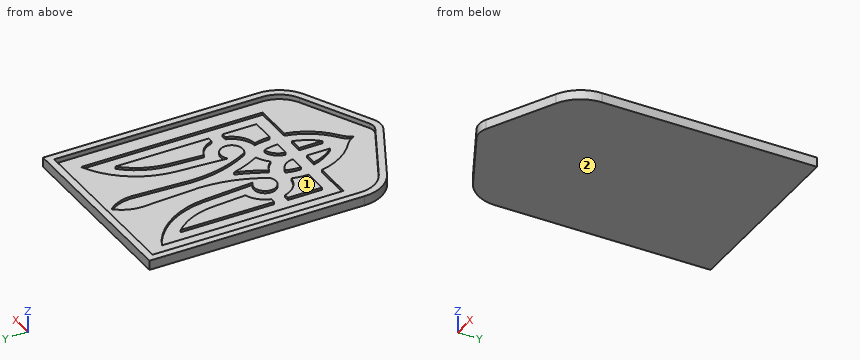
from build123d import *

# Parameters (mm, degrees)
EXTRUDE_1_DEPTH     = 2
EXTRUDE_2_DEPTH     = 2
OTHER_START         = 1
OTHER_1_DEPTH       = 1
CUT_EXTRUDE_1_DEPTH = 10


# Read off the part's stored shape, not the designer's step: Полость1
with BuildPart() as part:
    # Эскиз1 → Бобышка-Вытянуть1 (new body)
    with BuildSketch(Plane.XY):
        with BuildLine():
            Line((-3.59812982, 1.811928513), (-31.19625964, 15.709658955))
            ThreePointArc((-31.19625964, 15.709658955), (-37.622410841, 21.607746257), (-40, 30))
            Line((-40, 30), (-40, 120))
            Line((-40, 120), (40, 120))
            Line((40, 120), (40, 30))
            ThreePointArc((40, 30), (37.622410841, 21.607746257), (31.19625964, 15.709658955))
            Line((31.19625964, 15.709658955), (3.59812982, 1.811928513))
            ThreePointArc((3.59812982, 1.811928513), (0, 0.957099036), (-3.59812982, 1.811928513))
        make_face()
    extrude(amount=EXTRUDE_1_DEPTH)

    # Эскиз2 → Бобышка-Вытянуть2 (add)
    with BuildSketch(Plane.XY.offset(2)):
        with BuildLine():
            Line((40, 120), (-40, 120))
            Line((-40, 120), (-40, 30))
            ThreePointArc((-40, 30), (-37.622410841, 21.607746257), (-31.19625964, 15.709658955))
            Line((-31.19625964, 15.709658955), (-3.59812982, 1.811928513))
            ThreePointArc((-3.59812982, 1.811928513), (0, 0.957099036), (3.59812982, 1.811928513))
            Line((3.59812982, 1.811928513), (31.19625964, 15.709658955))
            ThreePointArc((31.19625964, 15.709658955), (37.622410841, 21.607746257), (40, 30))
            Line((40, 30), (40, 120))
        make_face()
        with BuildLine():
            Line((37, 117), (-37, 117))
            Line((-37, 117), (-37, 30))
            ThreePointArc((-37, 30), (-35.068208808, 23.181293834), (-29.846960958, 18.389097901))
            Line((-29.846960958, 18.389097901), (-2.248831138, 4.491367459))
            ThreePointArc((-2.248831138, 4.491367459), (0, 3.957099036), (2.248831138, 4.491367459))
            Line((2.248831138, 4.491367459), (29.846960958, 18.389097901))
            ThreePointArc((29.846960958, 18.389097901), (35.068208808, 23.181293834), (37, 30))
            Line((37, 30), (37, 117))
        make_face(mode=Mode.SUBTRACT)
    extrude(amount=EXTRUDE_2_DEPTH)

    # Полость1 outline → Полость1 (cut)
    with BuildSketch(Plane.XY.offset(OTHER_START)):
        with BuildLine():
            ThreePointArc((9.788029472, 60.549586915), (17.495233568, 56.130696454), (9.431968209, 52.400905625))
            ThreePointArc((9.431968209, 52.400905625), (4.262579544, 64.984556644), (2.5, 78.473966026))
            Line((2.5, 78.473966026), (3.75, 103.098966026))
            ThreePointArc((3.75, 103.098966026), (2.7812152, 108.402266884), (0, 113.020533442))
            ThreePointArc((0, 113.020533442), (-2.7812152, 108.402266884), (-3.75, 103.098966026))
            Line((-3.75, 103.098966026), (-2.5, 78.473966026))
            ThreePointArc((-2.5, 78.473966026), (-4.262579544, 64.984556644), (-9.431968209, 52.400905625))
            ThreePointArc((-9.431968209, 52.400905625), (-17.495233567, 56.130696454), (-9.788029472, 60.549586915))
            Line((-9.788029472, 60.549586915), (-11.224736233, 81.095450805))
            ThreePointArc((-11.224736233, 81.095450805), (-16.940759264, 97.456053222), (-30, 108.848966026))
            Line((-30, 108.848966026), (-30, 33.848966026))
            Line((-30, 33.848966026), (-13.791634566, 33.848966026))
            ThreePointArc((-13.791634566, 33.848966026), (-10.030008845, 24.210277963), (-2.972883984, 16.643830691))
            ThreePointArc((-2.972883984, 16.643830691), (-1.271172874, 15.008808512), (0, 13.020533442))
            ThreePointArc((0, 13.020533442), (1.271172874, 15.008808512), (2.972883984, 16.643830691))
            ThreePointArc((2.972883984, 16.643830691), (10.030008845, 24.210277963), (13.791634566, 33.848966026))
            Line((13.791634566, 33.848966026), (30, 33.848966026))
            Line((30, 33.848966026), (30, 108.848966026))
            ThreePointArc((30, 108.848966026), (16.940759264, 97.456053222), (11.224736233, 81.095450805))
            Line((11.224736233, 81.095450805), (9.788029472, 60.549586915))
        make_face()
        with BuildLine():
            ThreePointArc((-2.5, 22.780752061), (-6.389541147, 27.869966821), (-8.687410968, 33.848966026))
            Line((-8.687410968, 33.848966026), (-2.5, 33.848966026))
            Line((-2.5, 33.848966026), (-2.5, 22.780752061))
        make_face(mode=Mode.SUBTRACT)
        with BuildLine():
            ThreePointArc((-13.200536483, 46.373533772), (-13.986370475, 42.647666246), (-14.25, 38.848966026))
            Line((-14.25, 38.848966026), (-25, 38.848966026))
            Line((-25, 38.848966026), (-25, 53.848966026))
            Line((-25, 53.848966026), (-22.182458365, 53.848966026))
            ThreePointArc((-22.182458365, 53.848966026), (-18.897043641, 48.662755473), (-13.200536483, 46.373533772))
        make_face(mode=Mode.SUBTRACT)
        with BuildLine():
            ThreePointArc((-8.161111111, 45.763756043), (-3.92918135, 43.397470053), (-2.25, 38.848966026))
            Line((-2.25, 38.848966026), (-9.25, 38.848966026))
            ThreePointArc((-9.25, 38.848966026), (-8.976110771, 42.348966026), (-8.161111111, 45.763756043))
        make_face(mode=Mode.SUBTRACT)
        with BuildLine():
            Line((2.5, 22.780752061), (2.5, 33.848966026))
            Line((2.5, 33.848966026), (8.687410969, 33.848966026))
            ThreePointArc((8.687410969, 33.848966026), (6.389541147, 27.869966821), (2.5, 22.780752061))
        make_face(mode=Mode.SUBTRACT)
        with BuildLine():
            ThreePointArc((2.25, 38.848966026), (3.92918135, 43.397470053), (8.161111111, 45.763756043))
            ThreePointArc((8.161111111, 45.763756043), (8.976110771, 42.348966026), (9.25, 38.848966026))
            Line((9.25, 38.848966026), (2.25, 38.848966026))
        make_face(mode=Mode.SUBTRACT)
        with BuildLine():
            ThreePointArc((0, 63.756825508), (2.33883829, 56.831501462), (5.545675565, 50.262904017))
            ThreePointArc((5.545675565, 50.262904017), (2.504193555, 48.773385172), (0, 46.493408451))
            ThreePointArc((0, 46.493408451), (-2.504193555, 48.773385172), (-5.545675565, 50.262904017))
            ThreePointArc((-5.545675565, 50.262904017), (-2.33883829, 56.831501462), (0, 63.756825508))
        make_face(mode=Mode.SUBTRACT)
        with BuildLine():
            ThreePointArc((14.25, 38.848966026), (13.986370475, 42.647666246), (13.200536483, 46.373533772))
            ThreePointArc((13.200536483, 46.373533772), (18.897043642, 48.662755473), (22.182458366, 53.848966026))
            Line((22.182458366, 53.848966026), (25, 53.848966026))
            Line((25, 53.848966026), (25, 38.848966026))
            Line((25, 38.848966026), (14.25, 38.848966026))
        make_face(mode=Mode.SUBTRACT)
        with BuildLine():
            ThreePointArc((-15.180187421, 65.983103008), (-19.636717055, 63.353769354), (-22.182458365, 58.848966026))
            Line((-22.182458365, 58.848966026), (-25, 58.848966026))
            Line((-25, 58.848966026), (-25, 99.303564565))
            ThreePointArc((-25, 99.303564565), (-18.795712851, 90.606876243), (-16.177801663, 80.249651334))
            Line((-16.177801663, 80.249651334), (-15.180187421, 65.983103008))
        make_face(mode=Mode.SUBTRACT)
        with BuildLine():
            ThreePointArc((16.177801663, 80.249651334), (18.795712851, 90.606876243), (25, 99.303564565))
            Line((25, 99.303564565), (25, 58.848966026))
            Line((25, 58.848966026), (22.182458366, 58.848966026))
            ThreePointArc((22.182458366, 58.848966026), (19.636717055, 63.353769354), (15.180187421, 65.983103008))
            Line((15.180187421, 65.983103008), (16.177801663, 80.249651334))
        make_face(mode=Mode.SUBTRACT)
    extrude(amount=OTHER_1_DEPTH, mode=Mode.SUBTRACT)

    # Эскиз3 → Вырез-Вытянуть1 (cut)
    with BuildSketch(Plane.XY.offset(1)):
        with BuildLine():
            Line((-30.4, 109.485933086), (-30.4, 33.448966026))
            Line((-30.4, 33.448966026), (-14.122431386, 33.448966026))
            ThreePointArc((-14.122431386, 33.448966026), (-10.280405338, 23.857967906), (-3.211502278, 16.322782533))
            ThreePointArc((-3.211502278, 16.322782533), (-1.296555795, 14.391675131), (0, 12.001039461))
            ThreePointArc((0, 12.001039461), (1.296555795, 14.391675131), (3.211502278, 16.322782533))
            ThreePointArc((3.211502278, 16.322782533), (10.280405338, 23.857967906), (14.122431386, 33.448966026))
            Line((14.122431386, 33.448966026), (30.4, 33.448966026))
            Line((30.4, 33.448966026), (30.4, 109.485933086))
            ThreePointArc((30.4, 109.485933086), (16.789759987, 97.944057432), (10.825816986, 81.124874611))
            Line((10.825816986, 81.124874611), (9.326149592, 59.678631713))
            ThreePointArc((9.326149592, 59.678631713), (17.092035273, 56.619543276), (9.739143413, 52.669608621))
            ThreePointArc((9.739143413, 52.669608621), (4.640098892, 65.12142468), (2.900000984, 78.46383966))
            Line((2.900000984, 78.46383966), (4.149996614, 103.088753565))
            ThreePointArc((4.149996614, 103.088753565), (3.076851741, 108.747091307), (0, 113.615500626))
            ThreePointArc((0, 113.615500626), (-3.076851741, 108.747091307), (-4.149996614, 103.088753565))
            Line((-4.149996614, 103.088753565), (-2.900000984, 78.46383966))
            ThreePointArc((-2.900000984, 78.46383966), (-4.640098892, 65.12142468), (-9.739143413, 52.669608621))
            ThreePointArc((-9.739143413, 52.669608621), (-17.092035273, 56.619543276), (-9.326149592, 59.678631713))
            Line((-9.326149592, 59.678631713), (-10.825816986, 81.124874611))
            ThreePointArc((-10.825816986, 81.124874611), (-16.789759986, 97.944057431), (-30.4, 109.485933086))
        make_face()
        with BuildLine():
            Line((-24.6, 98.342803418), (-24.6, 59.248966026))
            Line((-24.6, 59.248966026), (-22.487492178, 59.248966026))
            ThreePointArc((-22.487492178, 59.248966026), (-19.927985451, 63.628047845), (-15.601624133, 66.275693973))
            Line((-15.601624133, 66.275693973), (-16.57694324, 80.223407018))
            ThreePointArc((-16.57694324, 80.223407018), (-18.961550559, 90.003486832), (-24.6, 98.342803418))
        make_face(mode=Mode.SUBTRACT)
        with BuildLine():
            Line((-24.6, 39.248966026), (-14.647132469, 39.248966026))
            ThreePointArc((-14.647132469, 39.248966026), (-14.388051735, 42.663162704), (-13.71270618, 46.019912646))
            ThreePointArc((-13.71270618, 46.019912646), (-19.220031201, 48.411637718), (-22.487492178, 53.448966026))
            Line((-22.487492178, 53.448966026), (-24.6, 53.448966026))
            Line((-24.6, 53.448966026), (-24.6, 39.248966026))
        make_face(mode=Mode.SUBTRACT)
        with BuildLine():
            Line((-8.846379794, 39.248966026), (-2.662132363, 39.248966026))
            ThreePointArc((-2.662132363, 39.248966026), (-4.251709751, 43.159081405), (-7.885555556, 45.306387443))
            ThreePointArc((-7.885555556, 45.306387443), (-8.577119532, 42.311169504), (-8.846379794, 39.248966026))
        make_face(mode=Mode.SUBTRACT)
        with BuildLine():
            Line((2.662132363, 39.248966026), (8.846379794, 39.248966026))
            ThreePointArc((8.846379794, 39.248966026), (8.577119532, 42.311169504), (7.885555556, 45.306387443))
            ThreePointArc((7.885555556, 45.306387443), (4.251709751, 43.159081405), (2.662132363, 39.248966026))
        make_face(mode=Mode.SUBTRACT)
        with BuildLine():
            Line((-2.9, 33.448966026), (-8.180118992, 33.448966026))
            ThreePointArc((-8.180118992, 33.448966026), (-6.154149081, 28.271206412), (-2.9, 23.762962579))
            Line((-2.9, 23.762962579), (-2.9, 33.448966026))
        make_face(mode=Mode.SUBTRACT)
        with BuildLine():
            Line((8.180118992, 33.448966026), (2.9, 33.448966026))
            Line((2.9, 33.448966026), (2.9, 23.762962579))
            ThreePointArc((2.9, 23.762962579), (6.154149081, 28.271206412), (8.180118992, 33.448966026))
        make_face(mode=Mode.SUBTRACT)
        with BuildLine():
            Line((14.647132469, 39.248966026), (24.6, 39.248966026))
            Line((24.6, 39.248966026), (24.6, 53.448966026))
            Line((24.6, 53.448966026), (22.487492178, 53.448966026))
            ThreePointArc((22.487492178, 53.448966026), (19.220031201, 48.411637718), (13.71270618, 46.019912646))
            ThreePointArc((13.71270618, 46.019912646), (14.388051735, 42.663162704), (14.647132469, 39.248966026))
        make_face(mode=Mode.SUBTRACT)
        with BuildLine():
            Line((22.487492178, 59.248966026), (24.6, 59.248966026))
            Line((24.6, 59.248966026), (24.6, 98.342803418))
            ThreePointArc((24.6, 98.342803418), (18.961550559, 90.003486832), (16.57694324, 80.223407018))
            Line((16.57694324, 80.223407018), (15.601624133, 66.275693973))
            ThreePointArc((15.601624133, 66.275693973), (19.927985451, 63.628047845), (22.487492178, 59.248966026))
        make_face(mode=Mode.SUBTRACT)
        with BuildLine():
            ThreePointArc((0, 47.107143791), (-2.273385478, 49.100153753), (-4.961500663, 50.483774724))
            ThreePointArc((-4.961500663, 50.483774724), (-2.150697128, 56.242155237), (0, 62.278218899))
            ThreePointArc((0, 62.278218899), (2.150697128, 56.242155237), (4.961500663, 50.483774724))
            ThreePointArc((4.961500663, 50.483774724), (2.273385478, 49.100153753), (0, 47.107143791))
        make_face(mode=Mode.SUBTRACT)
    extrude(amount=CUT_EXTRUDE_1_DEPTH, mode=Mode.SUBTRACT)


solid = part.part
Geometry: final body of the model. Coordinates: model frame, mm. Face numbers are marked on the shaded views. Coordinates: 2 decimals unless noted, no trailing zeros. Loops run counter-clockwise (first coordinate to the right, second up) from the corner with the lowest first, then second, coordinate; pieces in that order, holes last. Notation, with made-up numbers: (5.25, -26.5) - (19.25, -26.5) arc R24 ccw to (19.25, 4.5) - close; hole circle Ø6 at (66.5, 56.5). An arc over 180 degrees is marked (long way). One line per question, with ' | ' between items. Start each with the question number.
(1) Cut plane C-C on y = 71. Output: boundary loops of the cut face in (x, z), and give its area (3 significant figures).
(2) Cut plane D-D on x = 35. Output: boundary loops of the cut face in (y, z), and give its area (3 significant figures).
(3) First-contact query: pin 1 (1.6 mm diameter, centred on x = -5.5, y = 28, fed in from +Z); pin 2 (0.5 mm diameter, centred on y = 27, z = 1.5, fed in from -X); pin 3 (0.5 mm diameter, centred on x = 18.5, z = 1.5, fed in from -Y). Flat tips, straight axial feed; report the tip coordinate or a pass-through.
(4) Cut plane B-B on x = -12.5. Output: boundary loops of the cut face in (y, z), and give its area (3 significant figures).
(5) Ray query, L1, parallel to X at y = 67, z = 2.75; L2, parallel to Z at x = 29, y = 41; L3, parallel to Z at x = 36.5, y = 83.5. Return the intervals inside material, ascending. Write a range as from..to.
(6) Draft query along X for the marked faces 1 and 2. Return one class per face: +X half, -X half, draft (parallel to the pull), parting line (faces both ways), or undercut.
(7) Cut plane A-A on z = 3.4. Output: boundary loops of the cut face in (x, y).
Here are the results:
1) outline: (-40, 0) - (40, 0) - (40, 4) - (37, 4) - (37, 2) - (30.4, 2) - (30.4, 1) - (24.6, 1) - (24.6, 2) - (15.93, 2) - (15.93, 1) - (10.12, 1) - (10.12, 2) - (3.44, 2) - (3.44, 1) - (-3.44, 1) - (-3.44, 2) - (-10.12, 2) - (-10.12, 1) - (-15.93, 1) - (-15.93, 2) - (-24.6, 2) - (-24.6, 1) - (-30.4, 1) - (-30.4, 2) - (-37, 2) - (-37, 4) - (-40, 4) - close | area: 142 mm²
2) outline: (18.38, 0) - (120, 0) - (120, 4) - (117, 4) - (117, 2) - (23.07, 2) - (23.07, 4) - (18.38, 4) - close | area: 219 mm²
3) pin 1: z = 2 | pin 2: x = -39.76 | pin 3: y = 9.19
4) outline: (6.29, 0) - (120, 0) - (120, 4) - (117, 4) - (117, 2) - (89.37, 2) - (89.37, 1) - (60.95, 1) - (60.95, 2) - (51.75, 2) - (51.75, 1) - (28.11, 1) - (28.11, 2) - (9.65, 2) - (9.65, 4) - (6.29, 4) - close | area: 188 mm²
5) L1: -40..-37, 37..40 | L2: 0..1 | L3: 0..2
6) face 1: undercut | face 2: draft
7) outline: (-40, 30) arc R16 ccw to (-31.2, 15.71) - (-3.6, 1.81) arc R8 ccw to (3.6, 1.81) - (31.2, 15.71) arc R16 ccw to (40, 30) - (40, 120) - (-40, 120) - close; hole (-37, 30) arc R13 ccw to (-29.85, 18.39) - (-2.25, 4.49) arc R5 ccw to (2.25, 4.49) - (29.85, 18.39) arc R13 ccw to (37, 30) - (37, 117) - (-37, 117) - close
